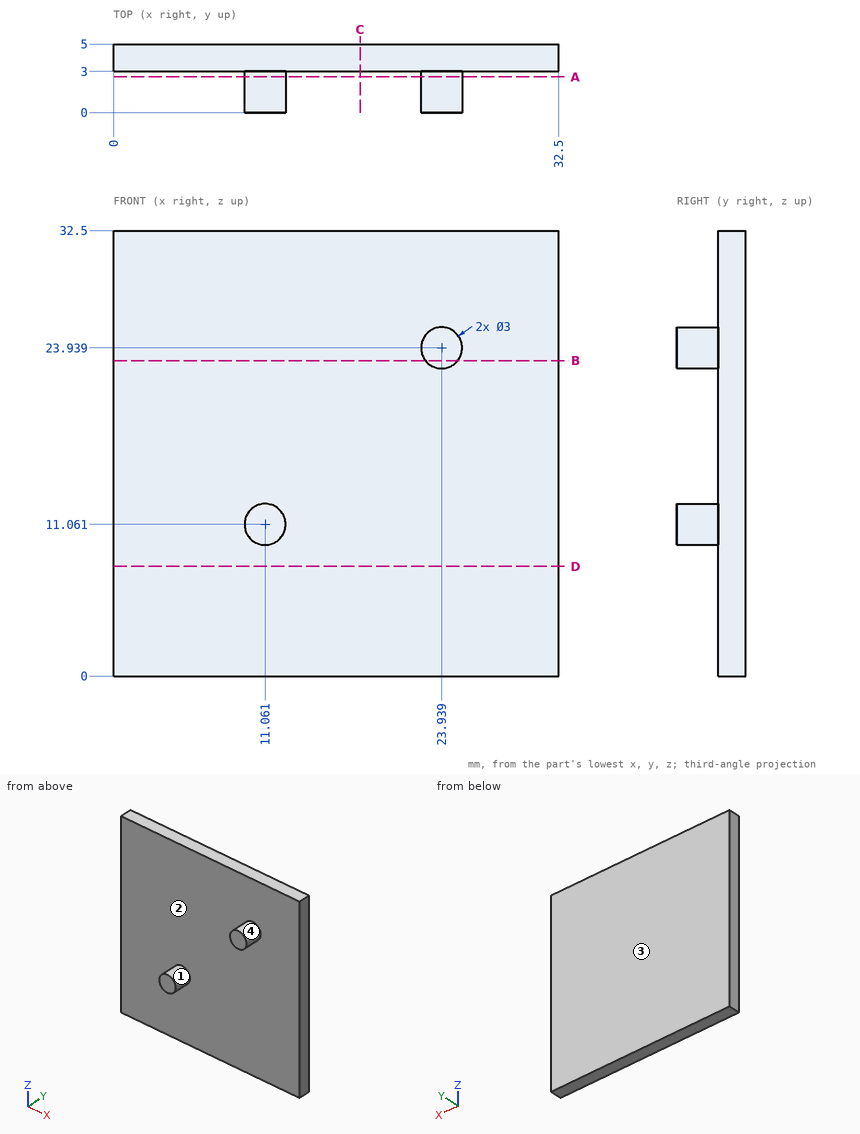
For this review, use the dimensioned drawing (mm, ordinates from the lowest corner) and the shaded views. A direction names the side the tool comes from. Round coordinates to 2 decimals unless told otherwise and drop trailing zeros. Write each loop counter-clockwise with the first axis right and the second up, starting at its lowest first coordinate (ties: lowest second). Pieces come first, ordered by that corner, then holes. Notation, with made-up numbers: (83, 89.5) - (89, 89.5) arc R7 ccw to (89, 93.5) - close; hole circle Ø11 at (64.25, 8.25). An arc over 180 degrees is marked (long way). Answer as a JSON object with one key per item and string values.
1. For pin 1 Ø6 at (x, z) = (14.5, 27) entering from -Y, flat-tipped, find the tip position at first contact; note if it passes through.
Response values:
{"pin 1": "stops at y = 3"}
2. We need section A-A on y = 2.6. Give the boundary of the cut face in (x, z), then the cut area to 3 significant figures.
Response values:
{"outline": "circle Ø3 at (11.06, 11.06); circle Ø3 at (23.94, 23.94)", "area": "14.1 mm2"}
3. We need section B-B on z = 23. Give the boundary of the cut face in (x, y).
Response values:
{"outline": "(0, 3) - (22.77, 3) - (22.77, 0) - (25.11, 0) - (25.11, 3) - (32.5, 3) - (32.5, 5) - (0, 5) - close"}
4. Draft analysis for pull direction X (two halves, no side actions). For the marked faces 1 and 2, state which applies: +X half, -X half, draft (parallel to the pull), parting line (faces both ways), or undercut.
Response values:
{"face 1": "parting line", "face 2": "draft"}
5. To check wall thickness, follow line 1 along Y through (x, z) = (8, 15); line 2 along Z through (x, y) = (10.5, 2.9). State the ranges of each line that lie inside material, in increasing order.
Response values:
{"line 1": "y = 3 to 5", "line 2": "z = 9.67 to 12.45"}
6. We need section D-D on z = 8. Give the boundary of the cut face in (x, y), then the cut area to 3 significant figures.
Response values:
{"outline": "(0, 3) - (32.5, 3) - (32.5, 5) - (0, 5) - close", "area": "65.0 mm2"}
7. Tool access review of the marked faces 3 and 4: name each direction out of +Z, -Z, +X, -X, +Y, -Y from which nothing blocks a thin tool from reaching the whole face with its end or side.
Response values:
{"face 3": "+Z, -Z, +X, -X, +Y", "face 4": "-Y"}
8. We need section C-C on x = 18. Give the boundary of the cut face in (y, z), then the cut area to 3 significant figures.
Response values:
{"outline": "(3, 0) - (5, 0) - (5, 32.5) - (3, 32.5) - close", "area": "65.0 mm2"}
